Could you check a few things on this drawing? It's one solid part, dimensions in mm from its lowest x, y, z. A direction names the side the tool comes from. Coordinates: 2 decimals unless noted, no trailing zeros. Order: outer loops, then holes, each group sorted by start corner. A loop starts at its lowest first (then second) coordinate and runs counter-clockwise, first axis right, second up.
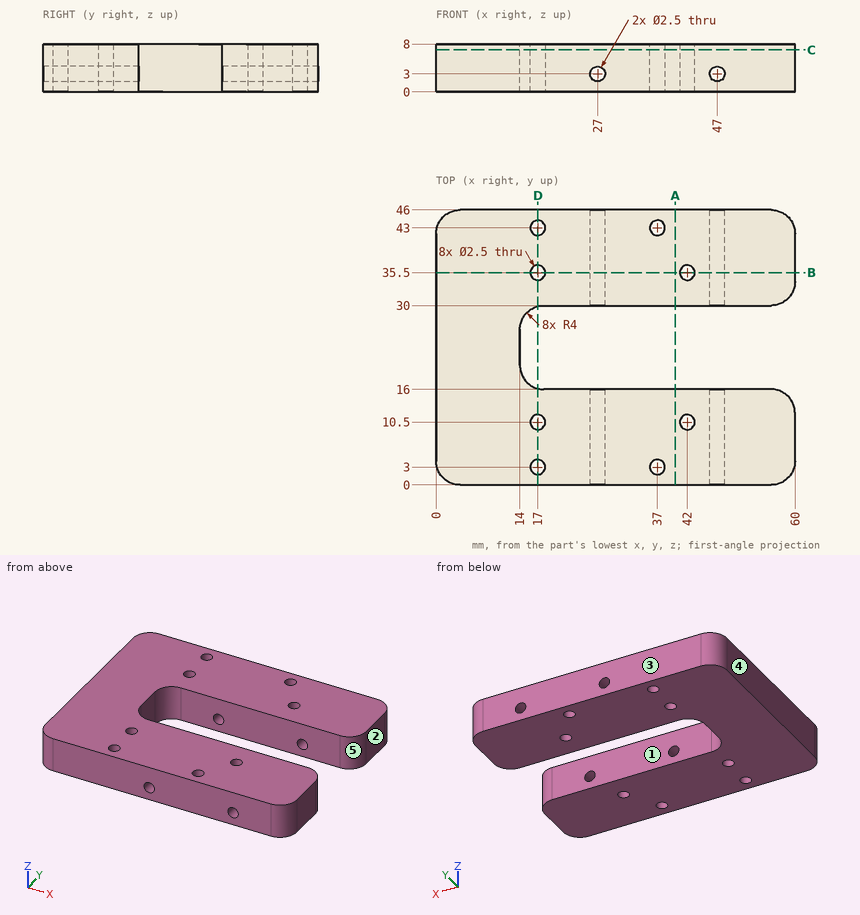
Q1. If we section it at B-B on y = 35.5: Write out the boundary of the cut face in (x, z), then the cut area to 3 significant figures.
Q2. If we section it at A-A on x = 40: Write out the boundary of the cut face in (y, z), then the cut area to 3 significant figures.
Q3. For the marked faces 4 and 5, which set-ups out of +Z, -Z, +X, -X, +Y, -Y let a thin tool reach every point of the face, with its end or its side?
Q4. If we section it at C-C on z = 7: Give the number of separate pieces and of enclosed holes in the cut face, then the cut area to 3 significant figures.
Q5. If we section it at D-D on x = 17: Write out the boundary of the cut face in (y, z), then the cut area to 3 significant figures.
Q6. I need wall thicknesses on L1, parallel to Y at x = 37, z = 5.25; L2, parallel to Y at x = 33, z = 6.25; L3, parallel to X at y = 12.5, z = 3. Which ranges of each line are inside material? Lowest first, please.
Q7. We'd pull the mould along Y, two halves only. Please class the marked faces 1, 2 and 3: pulls with the +Y half, pulls with the -Y half, needs draft (parallel to the pull), parting line crosses it, or undercut.
Reply:
1. outline: (0, 0) - (15.75, 0) - (15.75, 8) - (0, 8) - close; (18.25, 0) - (40.75, 0) - (40.75, 8) - (18.25, 8) - close; (43.25, 0) - (60, 0) - (60, 8) - (43.25, 8) - close; hole circle Ø2.5 at (27, 3); hole circle Ø2.5 at (47, 3)
1. area: 430 mm2
2. outline: (0, 0) - (16, 0) - (16, 8) - (0, 8) - close; (30, 0) - (46, 0) - (46, 8) - (30, 8) - close
2. area: 256 mm2
3. face 4: +Z, -Z, -X, +Y, -Y
3. face 5: +Z, -Z, +X
4. separate pieces: 1
4. enclosed holes: 8
4. area: 2,060 mm2
5. outline: (0, 0) - (1.75, 0) - (1.75, 8) - (0, 8) - close; (4.25, 0) - (9.25, 0) - (9.25, 8) - (4.25, 8) - close; (11.75, 0) - (16.13, 0) - (16.13, 8) - (11.75, 8) - close; (29.87, 0) - (34.25, 0) - (34.25, 8) - (29.87, 8) - close; (36.75, 0) - (41.75, 0) - (41.75, 8) - (36.75, 8) - close; (44.25, 0) - (46, 0) - (46, 8) - (44.25, 8) - close
5. area: 178 mm2
6. L1: y = 0 to 1.75, 4.25 to 16, 30 to 41.75, 44.25 to 46
6. L2: y = 0 to 16, 30 to 46
6. L3: x = 0 to 25.75, 28.25 to 45.75, 48.25 to 59.97
7. face 1: undercut
7. face 2: needs draft
7. face 3: pulls with the +Y half
